Input: part model. Units: mm. Frame: model coordinates. A direction names the side the tool comes from. Give positions to 0.01 mm unless a question says otherwise; leave off trailing zeros. Loops run counter-clockwise (first coordinate to the right, second up) from the corner with the lowest first, then second, coordinate; pieces in that order, holes last. Notation, with made-up numbers: M -4,29 L 36,29 A20 cw 36,65 Z; hole C 84,-36.5 d1. An arc over 180 degrees is marked long. Answer as a JSON object with one key per item and string values. Group by question number.
1) Ray query, L1, parallel to X at y = 13.25, z = 5.5; L2, parallel to Z at x = 16, y = 17.75. Return the intervals inside material, ascending.
2) First-contact query: P1, Ø5, axis at x = 12, y = 12.5, coming from the +Z side. Flat tip, straight axial feed; report the tip coordinate or a pass-through.
3) Access query for faces 1 (the flat face through (1, 10, 10)), 2 (the flat face through (18, 10, 6)). Directions: +Z, -Z, +X, -X, +Y, -Y. A direction counts if a zero-diameter tool reaches every point of the face in a straight line with its end or side. Return the directions, or none.
4) Section query B-B on y = 4.25. Return loops of the section in (x, z).
5) Draft query along X for faces 3 (the flat face through (2, 10, 6)), 4 (the flat face through (10, 20, 5)), 5 (the flat face through (0, 10, 5)). Return one class per face: +X half, -X half, draft (parallel to the pull), parting line (faces both ways), or undercut.
6) Section query A-A on z = 3.5. Return loops of the section in (x, y), plus the area to 3 significant figures.
from build123d import *

# Parameters (mm, degrees)
SKETCH_1_W    = 20
SKETCH_1_H    = 20
BASEBOX_DEPTH = 10
SHELL_T       = -2


with BuildPart() as part:
    # 草图1 → BaseBox (new body)
    with BuildSketch(Plane.XY):
        with Locations((10, 10)):
            Rectangle(SKETCH_1_W, SKETCH_1_H)
    extrude(amount=BASEBOX_DEPTH)

    # Shell
    shell_openings = [part.faces().sort_by_distance(p)[0] for p in [
        (10, 10, 10),
    ]]
    offset(amount=SHELL_T, openings=shell_openings, kind=Kind.INTERSECTION)


solid = part.part
Output:
{
 "1": {"L1": "x = 0 to 2, 18 to 20", "L2": "z = 0 to 2"},
 "2": {"P1": "stops at z = 2"},
 "3": {"face 1": "+Z, +X, -X, +Y, -Y", "face 2": "+Z"},
 "4": {"outline": "M 0,0 L 20,0 L 20,10 L 18,10 L 18,2 L 2,2 L 2,10 L 0,10 Z"},
 "5": {"face 3": "undercut", "face 4": "draft", "face 5": "-X half"},
 "6": {"outline": "M 0,0 L 20,0 L 20,20 L 0,20 Z; hole M 2,2 L 18,2 L 18,18 L 2,18 Z", "area": "144 mm^2"}
}
